Design review of the part built by this model. Coordinates are the model's own, in mm. Round coordinates to 2 decimals unless told otherwise and drop trailing zeros. Order: outer loops, then holes, each group sorted by start corner. A loop starts at its lowest first (then second) coordinate and runs counter-clockwise, first axis right, second up. Notation, with made-up numbers: (71.25, 19) - (104.25, 19) arc R10 ccw to (104.25, 34) - close; hole circle Ø6 at (61.5, 58.5). An arc over 180 degrees is marked (long way). Use CSV: the item, a comma, the result in double quotes. Start each with the question number.
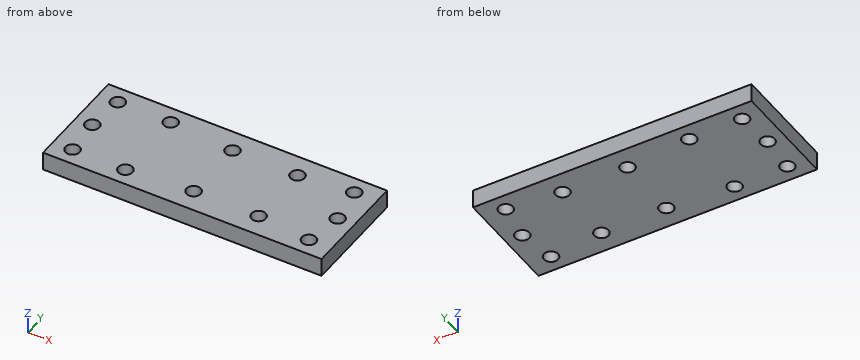
Autodesk Inventor part; units mm, degrees
ref_plane "YZ Plane" through (0, 0, 0) normal (1, 0, 0) x (0, 1, 0)
ref_plane "XZ Plane" through (0, 0, 0) normal (0, 1, 0) x (-1, 0, 0)
ref_plane "XY Plane" through (0, 0, 0) normal (0, 0, 1) x (1, 0, 0)
sketch "Esboço1" plane through (0, 0, 0) normal (0, 0, 1) x (1, 0, 0)
  line L0 (90, 0) -> (0, 0)
  line L1 (0, 0) -> (0, -35)
  line L2 (0, -35) -> (90, -35)
  line L3 (90, -35) -> (90, 0)
  circle A0 centre (65.3687, -7.1) radius 2.3
  circle A1 centre (23.3687, -29.5996) radius 2.3
  circle A2 centre (44.3687, -27.9) radius 2.3
  circle A3 centre (44.3687, -7.1) radius 2.3
  circle A4 centre (84.63, -17.5) radius 2.3
  circle A5 centre (5.3687, -17.5) radius 2.3
  circle A6 centre (65.3687, -27.9) radius 2.3
  circle A7 centre (23.3687, -5.4004) radius 2.3
  circle A8 centre (6.2932, -5.4004) radius 2.3
  circle A9 centre (6.2932, -29.5996) radius 2.3
  circle A10 centre (82.6841, -5.4004) radius 2.3
  circle A11 centre (82.6768, -29.5996) radius 2.3
extrude "Extrusão1" add sketch "Esboço1" along normal blind 6
properties part number "acrilico base" material "Acrílico"
Q1. Take a section at A-A (y = -17.5). State the section outline as (x, z) points, plus the area to 3 significant figures.
Q2. Take a section at B-B (x = 84). State the section outline as (y, z) points.
Q3. Clearance check with a flat-ended pin moving along its axis: pin 1 (6 mm diameter, centred on x = 23.37, y = -5.4, fed in from +Z). State where the tip first meets the part, or that it passes through.
Q4. For L1, parallel to Y at x = 45, z = 5.15; L2, parallel to Y at x = 46, z = 0.8; L3, parallel to X at y = -28, z = 2.8, list the stretches that pass through material, from the lowest coordinate up. Write a range as [from, to].
Q5. Take a section at C-C (z = 1). Give the number of separate pieces and of enclosed holes in the cut face, plus the area to 3 significant figures.
Findings below:
1,outline,"(0, 0) - (3.07, 0) - (3.07, 6) - (0, 6) - close; (7.67, 0) - (82.33, 0) - (82.33, 6) - (7.67, 6) - close; (86.93, 0) - (90, 0) - (90, 6) - (86.93, 6) - close"
1,area,"485 mm^2"
2,outline,"(-35, 0) - (-31.48, 0) - (-31.48, 6) - (-35, 6) - close; (-27.72, 0) - (-19.71, 0) - (-19.71, 6) - (-27.72, 6) - close; (-15.29, 0) - (-7.29, 0) - (-7.29, 6) - (-15.29, 6) - close; (-3.51, 0) - (0, 0) - (0, 6) - (-3.51, 6) - close"
3,pin 1,"stops at z = 6"
4,L1,"y = [-35, -30.11], [-25.69, -9.31], [-4.89, 0]"
4,L2,"y = [-35, -29.52], [-26.28, -8.72], [-5.48, 0]"
4,L3,"x = [0, 4.64], [7.95, 21.72], [25.02, 42.07], [46.67, 63.07], [67.67, 81.02], [84.33, 90]"
5,separate pieces,"1"
5,enclosed holes,"12"
5,area,"2,950 mm^2"
